CAD build for the part. Positions are in the model's coordinates, mm. Give positions to 0.01 mm unless a question says otherwise; leave off trailing zeros. Write each loop counter-clockwise with the first axis right and the second up, starting at its lowest first coordinate (ties: lowest second). Pieces come first, ordered by that corner, then holes. Notation, with made-up numbers: (-28.5, 17.25) - (-12.5, 17.25) arc R14 ccw to (-12.5, 41.25) - close; hole circle Ø4 at (-35, -27.75). An arc over 180 degrees is marked (long way). Answer as a JSON object with one key per item and string values.
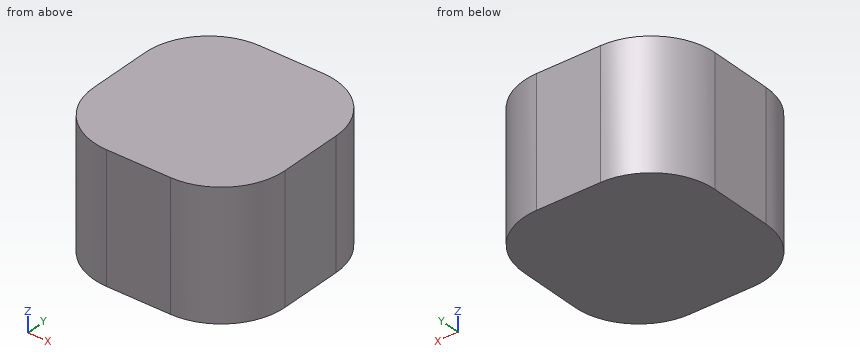
from build123d import *

# Parameters (mm, degrees)
F1_DEPTH = 76.2
F2_DEPTH = 25.4
F5_DEPTH = 50.8
F6_DEPTH = 25.4


with BuildPart() as f1:
    # F0 (on Top) → F1 (new body)
    with BuildSketch(Plane.XY):
        with BuildLine():
            ThreePointArc((31.75, 6.35), (28.0302561211, 15.3302561211), (19.05, 19.05))
            Line((19.05, 19.05), (-19.05, 19.05))
            ThreePointArc((-19.05, 19.05), (-28.0302561211, 15.3302561211), (-31.75, 6.35))
            Line((-31.75, 6.35), (-31.75, -6.35))
            ThreePointArc((-31.75, -6.35), (-28.0302561211, -15.3302561211), (-19.05, -19.05))
            Line((-19.05, -19.05), (19.05, -19.05))
            ThreePointArc((19.05, -19.05), (28.0302561211, -15.3302561211), (31.75, -6.35))
            Line((31.75, -6.35), (31.75, 6.35))
        make_face()
    extrude(amount=F1_DEPTH)

    # F2 (cut): a face of the model
    f2_faces = [f1.faces().sort_by_distance(p)[0] for p in [
        (0, 0, 76.2),
    ]]
    extrude(f2_faces, amount=-F2_DEPTH, mode=Mode.SUBTRACT)


with BuildPart() as f5:
    # F4 (on Top) → F5 (new body)
    with BuildSketch(Plane.XY):
        with BuildLine():
            Line((6.35, 19.05), (-6.35, 19.05))
            ThreePointArc((-6.35, 19.05), (-15.3302561211, 15.3302561211), (-19.05, 6.35))
            Line((-19.05, 6.35), (-19.05, -6.35))
            ThreePointArc((-19.05, -6.35), (-15.3302561211, -15.3302561211), (-6.35, -19.05))
            Line((-6.35, -19.05), (6.35, -19.05))
            ThreePointArc((6.35, -19.05), (15.3302561211, -15.3302561211), (19.05, -6.35))
            Line((19.05, -6.35), (19.05, 6.35))
            ThreePointArc((19.05, 6.35), (15.3302561211, 15.3302561211), (6.35, 19.05))
        make_face()
    extrude(amount=F5_DEPTH)

    # F6 (cut): a face of the model
    f6_faces = [f5.faces().sort_by_distance(p)[0] for p in [
        (0, 0, 50.8),
    ]]
    extrude(f6_faces, amount=-F6_DEPTH, mode=Mode.SUBTRACT)


solid = f5.part
(1) Flat gauge pins, fed straight in: P1, Ø2, axis at x = -10.5, z = 18, coming from the -Y side; P2, Ø12, axis at x = 11.5, y = -0.5, coming from the -Z side; P3, Ø5, axis at y = -13, z = 12.5, coming from the +X side; P4, Ø6, axis at x = -14, z = 21, coming from the +Y side. Where does each tip first touch, or does it go through?
Answer key:
{"P1": "stops at y = -18.65", "P2": "stops at z = 0", "P3": "stops at x = 18.35", "P4": "stops at y = 18.17"}
(2) Probe L1, parallel to Y at x = 13, z = 3.75; L2, parallel to X at y = -8, z = 9; L3, parallel to X at y = 11.5, z = 13.75. List the from-to ranges inside material, lowest first. Write a range as [from, to].
Answer key:
{"L1": "y = [-17.17, 17.17]", "L2": "x = [-18.94, 18.94]", "L3": "x = [-17.96, 17.96]"}
(3) Saw through at A-A, the plane z = 7.75. Give the cut face in (x, y), and give its area (3 significant figures).
Answer key:
{"outline": "(-19.05, -6.35) arc R12.7 ccw to (-6.35, -19.05) - (6.35, -19.05) arc R12.7 ccw to (19.05, -6.35) - (19.05, 6.35) arc R12.7 ccw to (6.35, 19.05) - (-6.35, 19.05) arc R12.7 ccw to (-19.05, 6.35) - close", "area": "1,310 mm²"}
(4) Saw through at C-C, the plane y = 13.5. Give the cut face in (x, z).
Answer key:
{"outline": "(-16.85, 0) - (16.85, 0) - (16.85, 25.4) - (-16.85, 25.4) - close"}
(5) Saw through at B-B, the plane x = -13. Give the cut face in (y, z), and give its area (3 significant figures).
Answer key:
{"outline": "(-17.17, 0) - (17.17, 0) - (17.17, 25.4) - (-17.17, 25.4) - close", "area": "872 mm²"}
